Work out the finished part from the listing and answer in its coordinate system (mm). A direction names the side the tool comes from. Round coordinates to 2 decimals unless told otherwise and drop trailing zeros. Order: outer loops, then holes, each group sorted by start corner. A loop starts at its lowest first (then second) coordinate and runs counter-clockwise, first axis right, second up. Notation, with made-up numbers: (40, -31) -> (96, -31) arc R16 cw to (96, -15) -> close; hole circle Ø1 at (61, -3.75). An arc over 180 degrees is marked (long way). Use one line per item in the form item = value.
```python
from build123d import *

# Parameters (mm, degrees)
SKETCH_1_W          = 85
SKETCH_1_H          = 56
SKETCH_1_R          = 1.5
EXTRUDE_1_DEPTH     = 2
SKETCH_2_W          = 10
SKETCH_2_H          = 10
EXTRUDE_2_DEPTH     = 2
SKETCH_3_W          = 10
SKETCH_3_H          = 21
EXTRUDE_3_DEPTH     = 10
SKETCH_4_W          = 5.6
SKETCH_4_H          = 2.2
CUT_EXTRUDE_1_DEPTH = 8
SKETCH_5_W          = 10
SKETCH_5_H          = 10
SKETCH_5_W_2        = 6
SKETCH_5_H_2        = 6
EXTRUDE_4_DEPTH     = 10
SKETCH_6_W          = 6
SKETCH_6_H          = 6
EXTRUDE_6_DEPTH     = 1
SKETCH_7_W          = 16
SKETCH_7_H          = 5
EXTRUDE_7_DEPTH     = 2


with BuildPart() as part:
    # 草图1 → 凸台-拉伸1 (new body)
    with BuildSketch(Plane(origin=(0, 0, 0), x_dir=(1, 0, 0), z_dir=(0, 1, 0))):
        Rectangle(SKETCH_1_W, SKETCH_1_H)
        with Locations(Location((-39, -24.5, 0), (0, 0, 270))):
            Circle(SKETCH_1_R, mode=Mode.SUBTRACT)
        with Locations(Location((-38.945993031, 24.5, 0), (0, 0, 270))):
            Circle(SKETCH_1_R, mode=Mode.SUBTRACT)
        with Locations(Location((19.054006969, 24.5, 0), (0, 0, 270))):
            Circle(SKETCH_1_R, mode=Mode.SUBTRACT)
        with Locations(Location((19.054006969, -24.5, 0), (0, 0, 270))):
            Circle(SKETCH_1_R, mode=Mode.SUBTRACT)
    extrude(amount=EXTRUDE_1_DEPTH)

    # 草图2 → 凸台-拉伸2 (add)
    with BuildSketch(Plane(origin=(0, 2, 0), x_dir=(1, 0, 0), z_dir=(0, 1, 0))):
        with Locations((-14.5, 0)):
            Rectangle(SKETCH_2_W, SKETCH_2_H)
    extrude(amount=EXTRUDE_2_DEPTH)

    # 草图3 → 凸台-拉伸3 (add)
    with BuildSketch(Plane(origin=(0, 2, 0), x_dir=(1, 0, 0), z_dir=(0, 1, 0))):
        with Locations((37.5, 12.5)):
            Rectangle(SKETCH_3_W, SKETCH_3_H)
    extrude(amount=EXTRUDE_3_DEPTH)

    # 草图4 → 切除-拉伸1 (cut)
    with BuildSketch(Plane(origin=(42.5, 0, 0), x_dir=(0, 0, -1), z_dir=(1, 0, 0))):
        with Locations((7.51, 7.9)):
            Rectangle(SKETCH_4_W, SKETCH_4_H)
        with Locations((7.51, 4.7)):
            Rectangle(SKETCH_4_W, SKETCH_4_H)
        with Locations((17.51, 7.9)):
            Rectangle(SKETCH_4_W, SKETCH_4_H)
        with Locations((17.6, 4.7)):
            Rectangle(SKETCH_4_W, SKETCH_4_H)
    extrude(amount=-CUT_EXTRUDE_1_DEPTH, mode=Mode.SUBTRACT)

    # 草图5 → 凸台-拉伸4 (add)
    with BuildSketch(Plane(origin=(42.5, 0, 0), x_dir=(0, 0, -1), z_dir=(1, 0, 0))):
        with Locations((-20, 7)):
            Rectangle(SKETCH_5_W, SKETCH_5_H)
        with Locations((-20, 7)):
            Rectangle(SKETCH_5_W_2, SKETCH_5_H_2, mode=Mode.SUBTRACT)
    extrude(amount=-EXTRUDE_4_DEPTH)

    # 草图6 → 凸台-拉伸6 (add)
    with BuildSketch(Plane.ZY.offset(-32.5)):
        with Locations((20, 7)):
            Rectangle(SKETCH_6_W, SKETCH_6_H)
    extrude(amount=-EXTRUDE_6_DEPTH)

    # 草图7 → 凸台-拉伸7 (add)
    with BuildSketch(Plane(origin=(0, 2, 0), x_dir=(1, 0, 0), z_dir=(0, 1, 0))):
        with Locations((-30.5, 16)):
            Rectangle(SKETCH_7_W, SKETCH_7_H)
    extrude(amount=EXTRUDE_7_DEPTH)


solid = part.part
```
Item 1: Consider line 1 along Y through (x, z) = (36, -19); line 2 along X through (y, z) = (1.4, -24.5); line 3 along Y through (x, z) = (-2.5, -1.5). Determine where each line is inside the solid, lowest interval first.
Findings:
line_1 = 0 to 3.6, 5.8 to 6.8, 9 to 12
line_2 = -42.5 to -40.45, -37.45 to 17.55, 20.55 to 42.5
line_3 = 0 to 2
Item 2: The part is cut by section C-C, the plane z = -24.5. Give the vertices of the cut face in (x, y), and give its area (3 significant figures).
Findings:
outline = (-42.5, 0) -> (-40.45, 0) -> (-40.45, 2) -> (-42.5, 2) -> close; (-37.45, 0) -> (17.55, 0) -> (17.55, 2) -> (-37.45, 2) -> close; (20.55, 0) -> (42.5, 0) -> (42.5, 2) -> (20.55, 2) -> close
area = 158 mm^2
Item 3: Flat-ended cylindrical pins translate along their axes: P1, Ø12, axis at x = 1, z = -3.5, coming from the +Y side; P2, Ø1.8, axis at x = 39.5, y = 8.5, coming from the +Z side; P3, Ø5, axis at x = 40, y = 8, coming from the -Z side. Find the tip coordinate at first contact, or state that the pin passes through.
Findings:
P1 = 2
P2 = 25
P3 = -23
Item 4: Determine the mould class of faces 4 (the flat face through (-38.5, 3, -16)), 5 (the flat face through (34.5, 8, -17)) for opening direction Y: released by +Y, released by -Y, zero draft, split by the parting line, or undercut.
Findings:
face_4 = zero draft
face_5 = undercut
Item 5: For faces 1 (the flat face through (32.5, 7, 20)), 2 (the flat face through (37, 7, -2)), 3 (the flat face through (39, 5, -20.4)), determine the directions among +Z, -Z, +X, -X, +Y, -Y from which every point of the face is accessible in a straight line to the end or side of a thin tool.
Findings:
face_1 = +Z, -Z, -X, +Y
face_2 = +X, +Y
face_3 = +X
Item 6: The part is cut by section B-B, the plane x = 37.5. Give the number of separate pieces and of enclosed holes in the cut face, and give its area (3 significant figures).
Findings:
separate_pieces = 1
enclosed_holes = 5
area = 337 mm^2
Item 7: The part is cut by section D-D, the plane x = 15.5. Give the vertices of the cut face in (y, z), and give its area (3 significant figures).
Findings:
outline = (0, -28) -> (2, -28) -> (2, 28) -> (0, 28) -> close
area = 112 mm^2
Item 8: The part is cut by section A-A, the plane y = 8. Give the vertices of the cut face in (x, z), and give its area (3 significant figures).
Findings:
outline = (32.5, -23) -> (42.5, -23) -> (42.5, -20.31) -> (34.5, -20.31) -> (34.5, -14.71) -> (42.5, -14.71) -> (42.5, -10.31) -> (34.5, -10.31) -> (34.5, -4.71) -> (42.5, -4.71) -> (42.5, -2) -> (32.5, -2) -> close; (32.5, 15) -> (42.5, 15) -> (42.5, 17) -> (33.5, 17) -> (33.5, 23) -> (42.5, 23) -> (42.5, 25) -> (32.5, 25) -> close
area = 166 mm^2
